```python
from build123d import *

# Parameters (mm, degrees)
BOSS_EXTRU_1_DEPTH      = 5
ENL_V_MAT_EXTRU_1_REACH = 110.282
ESQUISSE2_W             = 77
ESQUISSE2_H             = 21
ENL_V_MAT_EXTRU_2_REACH = 110.282
ESQUISSE4_R             = 1.5
ENL_V_MAT_EXTRU_3_DEPTH = 5


with BuildPart() as part:
    # Esquisse1 → Boss.-Extru.1 (new body)
    with BuildSketch(Plane.XY):
        Polygon((-90, 0), (90, 0), (90, 60), (-78.452994616, 60), (-90, 40), align=None)
    boss_extru_1 = extrude(amount=BOSS_EXTRU_1_DEPTH)

    # Symétrie1: Boss.-Extru.1 across Top Plane
    add(boss_extru_1.mirror(Plane(origin=(0, 0, 0), x_dir=(1, 0, 0), z_dir=(0, 1, 0))))

    # Esquisse2 → Enlèv. mat.-Extru.1 (cut, up to next)
    with BuildSketch(Plane.XY.offset(5), mode=Mode.PRIVATE) as enl_v_mat_extru_1_sk1:
        Rectangle(ESQUISSE2_W, ESQUISSE2_H)
    enl_v_mat_extru_1_tool1 = extrude(enl_v_mat_extru_1_sk1.sketch, amount=-ENL_V_MAT_EXTRU_1_REACH, mode=Mode.PRIVATE) & part.part
    add(enl_v_mat_extru_1_tool1.solids().sort_by_distance((0, 0, 5))[0], mode=Mode.SUBTRACT)

    # Esquisse3 → Enlèv. mat.-Extru.2 (cut, up to next)
    with BuildSketch(Plane.XY.offset(5), mode=Mode.PRIVATE) as enl_v_mat_extru_2_sk1:
        with BuildLine():
            Line((-38.5, 22.5), (38.5, 22.5))
            ThreePointArc((38.5, 22.5), (41, 20), (38.5, 17.5))
            Line((38.5, 17.5), (-38.5, 17.5))
            ThreePointArc((-38.5, 17.5), (-41, 20), (-38.5, 22.5))
        make_face()
    enl_v_mat_extru_2_tool1 = extrude(enl_v_mat_extru_2_sk1.sketch, amount=-ENL_V_MAT_EXTRU_2_REACH, mode=Mode.PRIVATE) & part.part
    enl_v_mat_extru_2 = enl_v_mat_extru_2_tool1.solids().sort_by_distance((0, 20, 5))[0]
    add(enl_v_mat_extru_2, mode=Mode.SUBTRACT)

    # Esquisse4 → Enlèv. mat.-Extru.3 (cut)
    with BuildSketch(Plane(origin=(0, 0, 0), x_dir=(-1, 0, 0), z_dir=(0, 0, -1))):
        with Locations((-75, 51.5)):
            Circle(ESQUISSE4_R)
        with Locations((8, 51.5)):
            Circle(ESQUISSE4_R)
        with Locations((70, 51.5)):
            Circle(ESQUISSE4_R)
        with Locations((-4, 27.5)):
            Circle(ESQUISSE4_R)
    enl_v_mat_extru_3 = extrude(amount=-ENL_V_MAT_EXTRU_3_DEPTH, mode=Mode.SUBTRACT)

    # Symétrie2: Enlèv. mat.-Extru.3 across plane
    add(enl_v_mat_extru_3.mirror(Plane.ZX), mode=Mode.SUBTRACT)

    # Symétrie3: Enlèv. mat.-Extru.2 across plane
    add(enl_v_mat_extru_2.mirror(Plane.ZX), mode=Mode.SUBTRACT)


solid = part.part
```
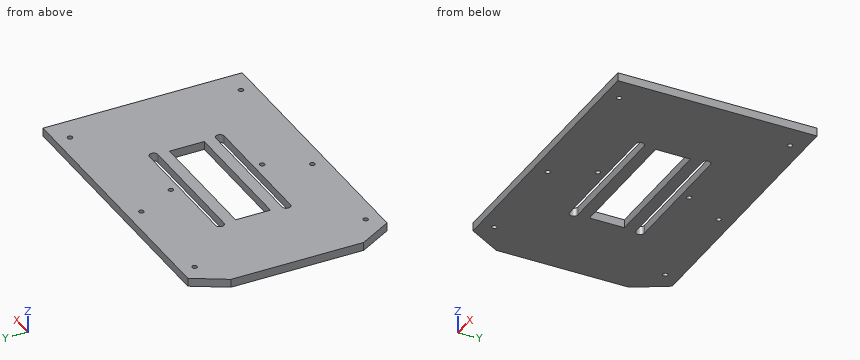
CAD build for the part. Positions are in the model's coordinates, mm. Coordinates: 2 decimals unless noted, no trailing zeros. Order: outer loops, then holes, each group sorted by start corner. A loop starts at its lowest first (then second) coordinate and runs counter-clockwise, first axis right, second up.
(1) Saw through at B-B, the plane y = 20. Write the cut outline in (x, z), and give its area (3 significant figures).
Solution:
outline: (-90, 0) - (-41, 0) - (-41, 5) - (-90, 5) - close; (41, 0) - (90, 0) - (90, 5) - (41, 5) - close
area: 490 mm2
(2) Saw through at A-A, the plane x = -33. Write the cut outline in (y, z), and give its area (3 significant figures).
Solution:
outline: (-60, 0) - (-22.5, 0) - (-22.5, 5) - (-60, 5) - close; (-17.5, 0) - (-10.5, 0) - (-10.5, 5) - (-17.5, 5) - close; (10.5, 0) - (17.5, 0) - (17.5, 5) - (10.5, 5) - close; (22.5, 0) - (60, 0) - (60, 5) - (22.5, 5) - close
area: 445 mm2
(3) Drill centre lines: L1, parallel to Y at x = 75, z = 2.85; L2, parallel to Y at x = 34, z = 2.1; L3, parallel to Y at x = 4, z = 1.6. Where is each one in solid material? Low to high.
Solution:
L1: y = -60 to -53, -50 to 50, 53 to 60
L2: y = -60 to -22.5, -17.5 to -10.5, 10.5 to 17.5, 22.5 to 60
L3: y = -60 to -29, -26 to -22.5, -17.5 to -10.5, 10.5 to 17.5, 22.5 to 26, 29 to 60
(4) Saw through at C-C, the plane z = 2.3. Count the separate pieces of the cut face and the enclosed holes in it, and give its area (3 significant figures).
Solution:
separate pieces: 1
enclosed holes: 11
area: 18,900 mm2
(5) Saw through at D-D, the plane y = -2. Write the cut outline in (x, z).
Solution:
outline: (-90, 0) - (-38.5, 0) - (-38.5, 5) - (-90, 5) - close; (38.5, 0) - (90, 0) - (90, 5) - (38.5, 5) - close
